Autodesk Inventor part; units mm, degrees
ref_plane "YZ Plane" through (0, 0, 0) normal (1, 0, 0) x (0, 1, 0)
ref_plane "XZ Plane" through (0, 0, 0) normal (0, 1, 0) x (-1, 0, 0)
ref_plane "XY Plane" through (0, 0, 0) normal (0, 0, 1) x (1, 0, 0)
sketch "Sketch1" plane through (0, 0, 0) normal (0, 1, 0) x (-1, 0, 0)
  line L0 (12.5, 5.5) -> (-12.5, 5.5)
  line L1 (-12.5, 5.5) -> (-12.5, -5.5)
  line L2 (-12.5, -5.5) -> (12.5, -5.5)
  line L3 (12.5, -5.5) -> (12.5, 5.5)
  line L4 (12.5, 5.5) -> (-12.5, -5.5) construction
  line L5 (-12.5, 5.5) -> (12.5, -5.5) construction
  point P0 (0, 0)
  dimension "d0" = 25
  dimension "d1" = 11
extrude "Extrusion1" add sketch "Sketch1" along normal blind 1.2
sketch "Sketch2" plane through (0, 1.2, 0) normal (0, 1, 0) x (1, 0, 0)
  line L0 (-12.5, 5.5) -> (12.5, 5.5)
  line L1 (12.5, 5.5) -> (12.5, 4.3)
  line L2 (12.5, 4.3) -> (-12.5, 4.3)
  line L3 (-12.5, 4.3) -> (-12.5, 5.5)
  line L4 (0, 4.3) -> (0, 1.8)
  line L5 (-12.5, 5.5) -> (-12.5, -5.5)
  line L6 (-12.5, 5.5) -> (-12.5, -5.5)
  line L7 (0, 0.6) -> (0, -4.3)
  line L8 (-12.5, -4.3) -> (12.5, -4.3)
  line L9 (12.5, -5.5) -> (12.5, -4.3)
  line L10 (-12.5, -4.3) -> (-12.5, -5.5)
  line L11 (-12.5, -5.5) -> (12.5, -5.5)
  line L12 (-2.4, 1.7967) -> (-2.4, 0.6)
  line L13 (-2.4, 0.6) -> (2.4, 0.6)
  line L14 (2.4, 0.6) -> (2.4, 1.7967)
  line L15 (-2.4, 1.7967) -> (2.4, 0.6) construction
  line L16 (-2.4, 0.6) -> (2.4, 1.7967) construction
  line L17 (-2.4, 1.7967) -> (-12.5, 1.7967)
  line L18 (-12.5, 0.6) -> (-12.5, 1.7967)
  line L19 (-12.5, 0.6) -> (-2.4, 0.6)
  line L20 (2.4, 1.7967) -> (12.5, 1.7967)
  line L21 (12.5, -5.5) -> (12.5, 5.5)
  line L22 (2.4, 0.6) -> (12.5, 0.6)
  line L23 (12.5, 0.6) -> (12.5, 1.7967)
  point P0 (0, 0)
  point P1 (0, 1.1983)
  dimension "d4" = 1.2
  dimension "d5" = 2.5
  dimension "d7" = 4.9
  dimension "d11" = 4.8
extrude "Extrusion2" add sketch "Sketch2" along normal blind 30 contours L0 L1 L2 L3 | L17 L12 L19 L5 | L21 L22 L14 L20 | L8 L9 L11 L5
fillet "Fillet1" radius 2 2 edges at (0, 1.2, 4.3) (0, 1.2, -4.3)
sketch "Sketch3" plane through (0, 31.2, 0) normal (0, 1, 0) x (1, 0, 0)
  line L0 (12.5, 5.5) -> (-12.5, 5.5)
  line L1 (0, 5.5) -> (0, 6.1)
  arc A0 (-12.5, 6.1) -> (12.5, 6.1) centre (0, 136.0083) ccw
  line L2 (-12.5, 6.1) -> (-12.5, 5.5)
  line L3 (12.5, 6.1) -> (12.5, 5.5)
  line L4 (-12.5, -5.5) -> (12.5, -5.5)
  line L5 (0, -5.5) -> (0, -6.1)
  arc A1 (-12.5, -5.5) -> (12.5, -5.5) centre (0, 124.4083) ccw
  point P0 (0, 0)
  dimension "d13" = 0.6
  dimension "d14" = 0.6
extrude "Extrusion3" add sketch "Sketch3" against normal blind 31.2
properties part number "HanesBand-Adjuster"
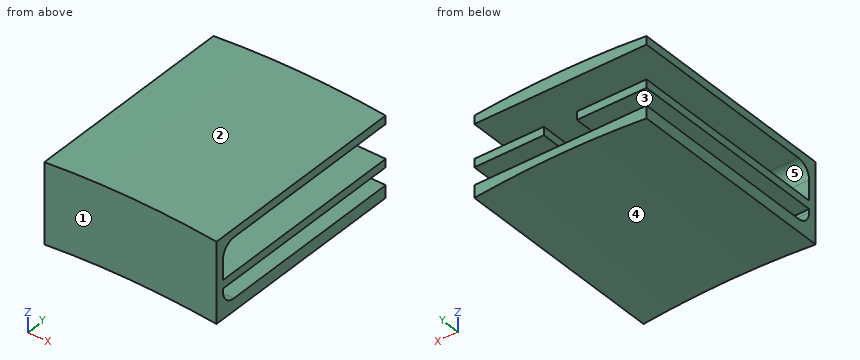
Geometry check sheet. Reference: the model listing, model coordinates, mm. Face numbers are marked on the shaded views. A direction names the side the tool comes from. Coordinates: 2 decimals unless noted, no trailing zeros. Order: outer loops, then holes, each group sorted by start corner. A loop starts at its lowest first (then second) coordinate and runs counter-clockwise, first axis right, second up. Notation, with made-up numbers: (82, -13.5) - (100, -13.5) arc R12 cw to (100, 4.5) - close; hole circle Ø5 at (-21.5, -33.75). An arc over 180 degrees is marked (long way). Answer as a JSON object with one key per item and string values. Group by question number.
Item 1: Sectioned sample at B-B, the plane z = 1.5. Record the cut outline in (x, y).
Item 2: Depth check by flat-ended pin: pin 1 Ø3 at (x, y) = (-8.5, 19) entering from -Z; pin 2 Ø3 at (x, y) = (-9.5, 20.5) entering from +Z; pin 3 Ø8 at (x, y) = (7, 15.5) entering from -Z. Enter the tip coordinate at first touch or a pass-through.
Item 3: Draft check along Z on the marked faces 1, 2 and 3. Enter one of: +Z half, -Z half, draft (parallel to the pull), parting line (faces both ways), or undercut.
Item 4: Sectioned sample at C-C, the plane x = 6.5. Record the cut outline in (y, z).
Item 5: Tool access check on the marked faces 4 and 5. Record the directions out of +Z, -Z, +X, -X, +Y, -Y that give a thin tool (end or side, any length) a straight path to the whole face; none if there is none.
Item 6: Sectioned sample at A-A, the plane y = 7.5. Record the cut outline in (x, z).
Item 7: Scan lines: probe 1 along Z at (x, y) = (0.25, 17); probe 2 along X at (y, z) = (2, -1.25); probe 3 along Z at (x, y) = (4.75, 4.5). Record each from-to range of solid material in increasing order.
Item 8: Sectioned sample at D-D, the plane x = 2. Record the cut outline in (y, z), and give its area (3 significant figures).
Resolved:
{
 "1": {"outline": "(-12.5, 0) - (12.5, 0) - (12.5, 1.2) - (-12.5, 1.2) - close"},
 "2": {"pin 1": "z = -5.88", "pin 2": "z = 5.85", "pin 3": "z = -5.96"},
 "3": {"face 1": "draft", "face 2": "+Z half", "face 3": "undercut"},
 "4": {"outline": "(0, -5.66) - (31.2, -5.66) - (31.2, -4.3) - (3.2, -4.3) arc R2 cw to (1.2, -2.3) - (1.2, -1.8) - (31.2, -1.8) - (31.2, -0.6) - (1.2, -0.6) - (1.2, 2.3) arc R2 cw to (3.2, 4.3) - (31.2, 4.3) - (31.2, 5.94) - (0, 5.94) - close"},
 "5": {"face 4": "-Z, +Y, -Y", "face 5": "+X, -X, +Y"},
 "6": {"outline": "(-12.5, -6.1) arc R130.51 cw to (12.5, -6.1) - (12.5, -4.3) - (-12.5, -4.3) - close; (-12.5, -1.8) - (-2.4, -1.8) - (-2.4, -0.6) - (-12.5, -0.6) - close; (-12.5, 4.3) - (12.5, 4.3) - (12.5, 5.5) arc R130.51 ccw to (-12.5, 5.5) - close; (2.4, -1.8) - (12.5, -1.8) - (12.5, -0.6) - (2.4, -0.6) - close"},
 "7": {"probe 1": "-5.5 to -4.3, 4.3 to 6.1", "probe 2": "-12.5 to -2.4, 2.4 to 12.5", "probe 3": "-5.59 to -4.3, -1.8 to -0.6, 4.3 to 6.01"},
 "8": {"outline": "(0, -5.52) - (31.2, -5.52) - (31.2, -4.3) - (3.2, -4.3) arc R2 cw to (1.2, -2.3) - (1.2, 2.3) arc R2 cw to (3.2, 4.3) - (31.2, 4.3) - (31.2, 6.08) - (0, 6.08) - close", "area": "106 mm^2"}
}
